```python
from build123d import *

# Parameters (mm, degrees)
F0_R     = 5.4
F1_DEPTH = 1
F2_R     = 9.25
F2_R_2   = 5.4
F3_DEPTH = 9
F4_R     = 1


with BuildPart() as f1:
    # F0 (on Top) → F1 (new body)
    with BuildSketch(Plane.XY):
        with BuildLine():
            ThreePointArc((25.1983354472, -0.625), (26.3689500386, -0.1587708172), (27.6189500386, 0))
            Line((27.6189500386, 0), (100.3810499614, 0))
            ThreePointArc((100.3810499614, 0), (101.6310499614, -0.1587708172), (102.8016645528, -0.625))
            ThreePointArc((102.8016645528, -0.625), (130.6811062012, 12.5335506494), (109.3784879352, 34.8182803278))
            Line((109.3784879352, 34.8182803278), (96.9014291121, 40.5587357108))
            ThreePointArc((96.9014291121, 40.5587357108), (92.9828428426, 42.4600025358), (88.6335206854, 42.691369483))
            Line((88.6335206854, 42.691369483), (25.4897410073, 33.3968526715))
            ThreePointArc((25.4897410073, 33.3968526715), (24.1939378933, 33.3758798492), (22.936271789, 33.688644201))
            ThreePointArc((22.936271789, 33.688644201), (-2.9588483895, 14.7501729139), (25.1983354472, -0.625))
        make_face()
        with Locations((90.2354166667, 31.8086341069)):
            Circle(F0_R, mode=Mode.SUBTRACT)
    extrude(amount=F1_DEPTH)

    # F2 (on face) → F3 (join)
    with BuildSketch(Plane(origin=(0, 0, 0), x_dir=(1, 0, 0), z_dir=(0, 0, -1))):
        with Locations((90.2354166667, -31.8086341069)):
            Circle(F2_R)
        with Locations((90.2354166667, -31.8086341069)):
            Circle(F2_R_2, mode=Mode.SUBTRACT)
    extrude(amount=F3_DEPTH)

    # F4
    f4_edges = [f1.edges().sort_by_distance(p)[0] for p in [
        (80.985417, 31.808634, -9),
        (84.835417, 31.808634, 1),
    ]]
    fillet(f4_edges, radius=F4_R)


solid = f1.part
```
The listing builds one solid part. Answer for the finished solid, in the listing's coordinates (mm). A direction names the side the tool comes from. Give positions to 0.01 mm unless a question says otherwise; leave off trailing zeros. Order: outer loops, then holes, each group sorted by start corner. A loop starts at its lowest first (then second) coordinate and runs counter-clockwise, first axis right, second up.
1) Find section B-B on y = 16. Write down the section's boundary in (x, z).
Reported:
outline: (-3, 0) - (131, 0) - (131, 1) - (-3, 1) - close
2) Given P1, Ø5, axis at y = 23.5, z = -5.5, coming from the -X side; P2, Ø5, axis at x = 46, y = 2, coming from the -Z side; P3, Ø0.5, axis at x = 76.5, z = 0.5, coming from the -Y side, each flat-ended and moving along its own axis, determine where each tip first touches the part or whether it passes through.
Reported:
P1: stops at x = 83.04
P2: stops at z = 0
P3: stops at y = 0
3) Determine the mould class of faces 3 (the face through (63, 20, 1)), 4 (the face through (93.042, 42.445, 0.493)), 5 (the face through (95.224, 33.877, -4.437)) for opening direction Y: pulls with the +Y half, pulls with the -Y half, needs draft (parallel to the pull), parting line crosses it, or undercut.
Reported:
face 3: needs draft
face 4: pulls with the +Y half
face 5: undercut
4) Find section C-C on x = 112. Write down the section's boundary in (y, z), then the cut area to 3 significant figures.
Reported:
outline: (-3, 0) - (35, 0) - (35, 1) - (-3, 1) - close
area: 38.0 mm2
5) Find section A-A on z = -6. Write down the section's boundary in (x, y).
Reported:
outline: circle Ø18.5 at (90.24, 31.81); hole circle Ø10.8 at (90.24, 31.81)
6) Consider line 1 along Z through (x, y) = (38, 22.5); line 2 along X through (y, z) = (36, -6.25); line 3 along Y through (x, z) = (98, 0.25). Determine where each line is inside the solid, lowest interval first.
Reported:
line 1: z = 0 to 1
line 2: x = 81.99 to 86.83, 93.64 to 98.48
line 3: y = 0 to 40.05
7) For faces 1 (the face through (96, 34, -9)), 2 (the face through (98.78, 35.35, -3.94)), determine the directions among +Z, -Z, +X, -X, +Y, -Y from which every point of the face is accessible in a straight line to the end or side of a thin tool.
Reported:
face 1: -Z, +X, -X, +Y, -Y
face 2: -Z
